Check sheet for the modelled part. Datum: model origin and axes. Units: mm. Face numbers are marked on the shaded views. A direction names the side the tool comes from. Round coordinates to 2 decimals unless told otherwise and drop trailing zeros. Write each loop counter-clockwise with the first axis right and the second up, starting at its lowest first coordinate (ties: lowest second). Pieces come first, ordered by that corner, then holes. Notation, with made-up numbers: (43, -26.5) - (75, -26.5) arc R13 ccw to (75, -10.5) - close; hole circle Ø7 at (60.5, -26). An arc over 180 degrees is marked (long way). Use one line per item in the form item = value. Start each with the question number.
1) Scan lines: probe 1 along X at (y, z) = (1.5, -2); probe 2 along Y at (x, z) = (26, 16.5); probe 3 along Y at (x, z) = (24.5, -27.5). Record each from-to range of solid material in increasing order.
2) Set-up check for the marked faces 1 and 2: record each of +Z, -Z, +X, -X, +Y, -Y from which the full face is reachable in a straight line by a thin tool's end or side.
3) Section check B-B (y = -105). Record the boundary of the cut face in (x, z), then the cut area to 3 significant figures.
4) Gauge pin test, flat ends, axial feed: P1, Ø12, axis at x = 14.5, y = 61.5, coming from the -Z side; P2, Ø5, axis at y = -8.5, z = -24.5, coming from the -X side; P3, Ø4, axis at y = -38, z = -20, coming from the -X side. Record the tip position at first contact, or that the pin passes through.
5) Section check A-A (y = -49). Record the boundary of the cut face in (x, z), then the cut area to 3 significant figures.
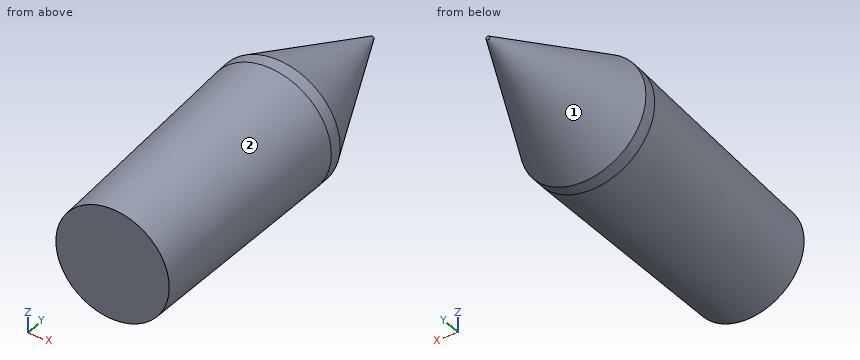
from build123d import *

# Parameters (mm, degrees)
F1_R      = 42.291
F2_R      = 38.0365
F4_DEPTH  = 8.636
F4_FACE_R = 42.291
F6_R      = 1.27


with BuildPart() as f3:
    # F1 (on Front) → F3 section 0
    with BuildSketch(Plane.XZ):
        Circle(F1_R)
    # F2 (on offset) → F3 section 1
    with BuildSketch(Plane.XZ.offset(152.4)):
        Circle(F2_R)
    loft()

    # F4 (add): a face of the model
    f4_faces = [f3.faces().sort_by_distance(p)[0] for p in [
        (0, 0, 0),
    ]]
    extrude(f4_faces, amount=F4_DEPTH)

    # F4_face (on face) → F7 section 0
    with BuildSketch(Plane(origin=(0, 8.636, 0), x_dir=(-1, 0, 0), z_dir=(0, 1, 0))):
        Circle(F4_FACE_R)
    # F6 (on offset) → F7 section 1
    with BuildSketch(Plane.XZ.offset(-101.6)):
        Circle(F6_R)
    loft()


solid = f3.part
Results are:
q1.probe_1 = -42.24 to 42.24
q1.probe_2 = -152.4 to 34.69
q1.probe_3 = -152.4 to 21.01
q2.face_1 = +Y
q2.face_2 = -Y
q3.outline = circle Ø78.72 at (0, 0)
q3.area = 4,870 mm²
q4.P1 = -18.14
q4.P2 = -35.84
q4.P3 = -37.1
q5.outline = circle Ø81.85 at (0, 0)
q5.area = 5,260 mm²
